```python
from build123d import *

# Parameters (mm, degrees)
SKETCH_W     = 228
SKETCH_H     = 130
SKETCH_R     = 1.75
PAD_DEPTH    = 3
SKETCH001_W  = 5
SKETCH001_H  = 120
PAD001_DEPTH = 10
SKETCH002_R  = 1.15
SKETCH002_W  = 95
SKETCH002_H  = 4
POCKET_DEPTH = 225


with BuildPart() as part:
    # Sketch → Pad (new body)
    with BuildSketch(Plane.XY):
        with Locations((-4, 0)):
            Rectangle(SKETCH_W, SKETCH_H)
        with Locations((-90, 62)):
            Circle(SKETCH_R, mode=Mode.SUBTRACT)
        with Locations((0, 62)):
            Circle(SKETCH_R, mode=Mode.SUBTRACT)
        with Locations((90, 62)):
            Circle(SKETCH_R, mode=Mode.SUBTRACT)
        with Locations((-90, -62)):
            Circle(SKETCH_R, mode=Mode.SUBTRACT)
        with Locations((0, -62)):
            Circle(SKETCH_R, mode=Mode.SUBTRACT)
        with Locations((90, -62)):
            Circle(SKETCH_R, mode=Mode.SUBTRACT)
        with BuildLine():
            ThreePointArc((10.059248, 43.499956), (8.309248, 41.749956), (10.059248, 39.999956))
            Line((10.059248, 39.999956), (90.059248, 39.999956))
            ThreePointArc((90.059248, 39.999956), (91.809248, 41.749956), (90.059248, 43.499956))
            Line((10.059248, 43.499956), (90.059248, 43.499956))
        make_face(mode=Mode.SUBTRACT)
        with BuildLine():
            ThreePointArc((10.044436, 33.499967), (8.294436, 31.749967), (10.044436, 29.999967))
            Line((10.044436, 29.999967), (90.044436, 29.999967))
            ThreePointArc((90.044436, 29.999967), (91.794436, 31.749967), (90.044436, 33.499967))
            Line((10.044436, 33.499967), (90.044436, 33.499967))
        make_face(mode=Mode.SUBTRACT)
        with BuildLine():
            ThreePointArc((10.029624, 23.499978), (8.279624, 21.749978), (10.029624, 19.999978))
            Line((10.029624, 19.999978), (90.029624, 19.999978))
            ThreePointArc((90.029624, 19.999978), (91.779624, 21.749978), (90.029624, 23.499978))
            Line((10.029624, 23.499978), (90.029624, 23.499978))
        make_face(mode=Mode.SUBTRACT)
        with BuildLine():
            ThreePointArc((10.014812, 13.499989), (8.264812, 11.749989), (10.014812, 9.999989))
            Line((10.014812, 9.999989), (90.014812, 9.999989))
            ThreePointArc((90.014812, 9.999989), (91.764812, 11.749989), (90.014812, 13.499989))
            Line((10.014812, 13.499989), (90.014812, 13.499989))
        make_face(mode=Mode.SUBTRACT)
        with BuildLine():
            ThreePointArc((10, 3.5), (8.25, 1.75), (10, 0))
            Line((10, 0), (90, 0))
            ThreePointArc((90, 0), (91.75, 1.75), (90, 3.5))
            Line((10, 3.5), (90, 3.5))
        make_face(mode=Mode.SUBTRACT)
    extrude(amount=PAD_DEPTH)

    # Sketch001 → Pad001 (join)
    with BuildSketch(Plane.XY.offset(3)):
        with Locations((104.5, 5)):
            Rectangle(SKETCH001_W, SKETCH001_H)
        with Locations((-104.5, 5)):
            Rectangle(SKETCH001_W, SKETCH001_H)
    extrude(amount=PAD001_DEPTH)

    # Sketch002 → Pocket (cut)
    with BuildSketch(Plane.YZ.offset(107)):
        with Locations((-51, 7)):
            Circle(SKETCH002_R)
        with Locations((61, 7)):
            Circle(SKETCH002_R)
        with Locations((7.5, 11)):
            Rectangle(SKETCH002_W, SKETCH002_H)
    extrude(amount=-POCKET_DEPTH, mode=Mode.SUBTRACT)


solid = part.part
```
Source: CAD feature listing. Evaluate the final solid. Frame: model axes, mm. A direction names the side the tool comes from. Coordinates: 2 decimals unless noted, no trailing zeros. Write each loop counter-clockwise with the first axis right and the second up, starting at its lowest first coordinate (ties: lowest second). Pieces come first, ordered by that corner, then holes. Notation, with made-up numbers: (87.25, 62.5) - (135.25, 62.5) arc R27 ccw to (135.25, 84.5) - close; hole circle Ø5 at (40.25, 7.25). An arc over 180 degrees is marked (long way). Answer as a JSON object with one key per item and string values.
Q1. Set-up query: faces 4 (the flat face through (-107, 4, 7)), 5 (the flat face through (-105, -55, 8)), 6 (the flat face through (-102, 4, 7)). Return all of +Z, -Z, +X, -X, +Y, -Y with unobstructed straight access to the full face (end or side cutting, diameter ignored); none if empty.
Ans:
{"face 4": "+Z, -X, +Y, -Y", "face 5": "+Z, +X, -X, -Y", "face 6": "+Z, +Y, -Y"}
Q2. Section query C-C, the plane x = -57. Output: boundary loops of the cut face in (y, z), plus the area to 3 significant figures.
Ans:
{"outline": "(-65, 0) - (65, 0) - (65, 3) - (-65, 3) - close", "area": "390 mm2"}
Q3. Draft query along X for faces 1 (the flat face through (105, -40, 11)), 2 (the flat face through (107, 4, 7)), 3 (the flat face through (102, 4, 7)). Return one class per face: released by +X, released by -X, zero draft, split by the parting line, or undercut.
Ans:
{"face 1": "zero draft", "face 2": "released by +X", "face 3": "undercut"}
Q4. Section query A-A, the plane x = 80.5. Output: boundary loops of the cut face in (y, z).
Ans:
{"outline": "(-65, 0) - (0, 0) - (0, 3) - (-65, 3) - close; (3.5, 0) - (10, 0) - (10, 3) - (3.5, 3) - close; (13.5, 0) - (20, 0) - (20, 3) - (13.5, 3) - close; (23.5, 0) - (30, 0) - (30, 3) - (23.5, 3) - close; (33.5, 0) - (40, 0) - (40, 3) - (33.5, 3) - close; (43.5, 0) - (65, 0) - (65, 3) - (43.5, 3) - close"}
Q5. Material intervals for line 1 (Y direction, x = -90, z = 0.8); line 2 (X direction, y = 53, z = 6.25); line 3 (Z direction, x = -104, y = -51), sorted ascending. Write a range as [from, to].
Ans:
{"line 1": "y = [-65, -63.75], [-60.25, 60.25], [63.75, 65]", "line 2": "x = [-107, -102], [102, 107]", "line 3": "z = [0, 5.85], [8.15, 13]"}
Q6. Section query B-B, the plane y = -22. Output: boundary loops of the cut face in (x, z).
Ans:
{"outline": "(-118, 0) - (110, 0) - (110, 3) - (107, 3) - (107, 9) - (102, 9) - (102, 3) - (-102, 3) - (-102, 9) - (-107, 9) - (-107, 3) - (-118, 3) - close"}
Q7. First-contact query: pin 1 Ø8 at (x, y) = (-41.5, 48.5) entering from +Z; pin 2 Ø5.5 at (x, y) = (105.5, 11.5) entering from +Z; pin 3 Ø3 at (x, y) = (0, -62) entering from -Z; pin 4 Ø5.5 at (x, z) = (-104.5, 6) entering from -Y. Flat tips, straight axial feed; report the tip coordinate or a pass-through.
Ans:
{"pin 1": "stops at z = 3", "pin 2": "stops at z = 9", "pin 3": "passes through", "pin 4": "stops at y = -55"}
